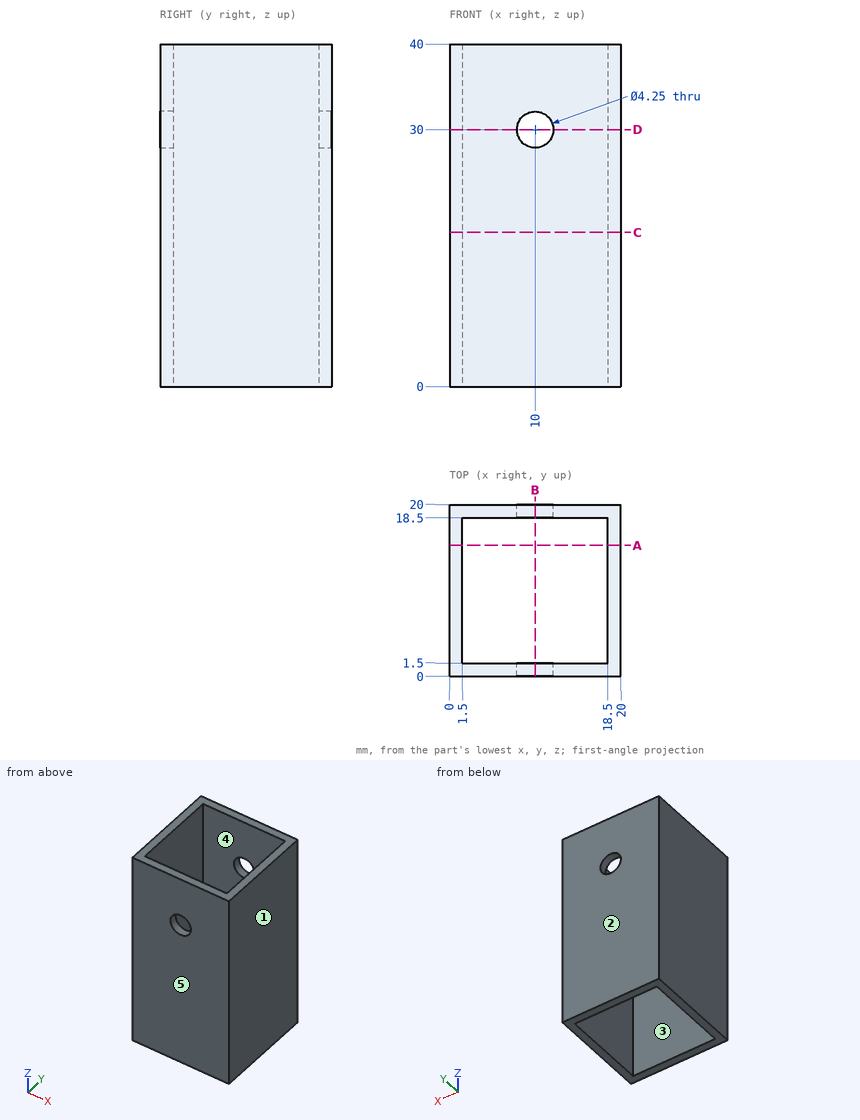
Job drawing, mm, ordinate dimensions from the low corner. One solid piece. A direction names the side the tool comes from. Coordinates: 2 decimals unless noted, no trailing zeros. Loops run counter-clockwise (first coordinate to the right, second up) from the corner with the lowest first, then second, coordinate; pieces in that order, holes last. Notation, with made-up numbers: (-21, 41) -> (30, 41) arc R12 cw to (30, 53) -> close; hole circle Ø6 at (-27, 10.25). An arc over 180 degrees is marked (long way). One line per item, written item: value.
1. Slice it at A-A on y = 15.25. Write the cut outline in (x, z).
Answers:
outline: (0, 0) -> (1.5, 0) -> (1.5, 40) -> (0, 40) -> close; (18.5, 0) -> (20, 0) -> (20, 40) -> (18.5, 40) -> close
2. Slice it at C-C on z = 18. Write the cut outline in (x, y), and give its area (3 significant figures).
Answers:
outline: (0, 0) -> (20, 0) -> (20, 20) -> (0, 20) -> close; hole (1.5, 1.5) -> (18.5, 1.5) -> (18.5, 18.5) -> (1.5, 18.5) -> close
area: 111 mm^2
3. Which spindle directions (+Z, -Z, +X, -X, +Y, -Y) get a long thin tool onto all of the face, cutting with end or side? Do the marked faces 4 and 5. Say none if no direction does.
Answers:
face 4: +Z, -Z
face 5: +Z, -Z, +X, -X, -Y
4. Slice it at D-D on z = 30. Write the cut outline in (x, y) (3 decimals), and give its area (4 significant figures).
Answers:
outline: (0, 0) -> (7.875, 0) -> (7.875, 1.5) -> (1.5, 1.5) -> (1.5, 18.5) -> (7.875, 18.5) -> (7.875, 20) -> (0, 20) -> close; (12.125, 0) -> (20, 0) -> (20, 20) -> (12.125, 20) -> (12.125, 18.5) -> (18.5, 18.5) -> (18.5, 1.5) -> (12.125, 1.5) -> close
area: 98.25 mm^2
5. Slice it at B-B on x = 10. Write the cut outline in (y, z) (3 decimals).
Answers:
outline: (0, 0) -> (1.5, 0) -> (1.5, 27.875) -> (0, 27.875) -> close; (0, 32.125) -> (1.5, 32.125) -> (1.5, 40) -> (0, 40) -> close; (18.5, 0) -> (20, 0) -> (20, 27.875) -> (18.5, 27.875) -> close; (18.5, 32.125) -> (20, 32.125) -> (20, 40) -> (18.5, 40) -> close
6. Drill centre lines: line 1 (Y direction, x = 7.25, z = 31.5); line 2 (X direction, y = 1.1, z = 30) (3 decimals). Where is each one in solid material? Low to high. Write a range as [from, to].
Answers:
line 1: y = [0, 1.5], [18.5, 20]
line 2: x = [0, 7.875], [12.125, 20]
7. Pull direction Y, two halves, no side cores. Call the marked faces 1, 2 and 3: pulls with the +Y half, pulls with the -Y half, needs draft (parallel to the pull), parting line crosses it, or undercut.
Answers:
face 1: needs draft
face 2: pulls with the +Y half
face 3: undercut
8. Flat gauge pin, fed straight in: P1, Ø10, axis at x = 10.5, y = 7.5, coming from the +Z side. Where does the tip first touch, or does it go through?
Answers:
P1: passes through
